Geometry: final body of the model. Coordinates: model frame, mm. A direction names the side the tool comes from. Give positions to 0.01 mm unless a question says otherwise; leave off trailing zeros. Write each loop counter-clockwise with the first axis right and the second up, starting at its lowest first coordinate (ties: lowest second). Pieces come first, ordered by that corner, then holes.
from build123d import *

# Parameters (mm, degrees)
F0_R     = 10.936503
F1_DEPTH = 7.0104
F2_R     = 10.16
F3_R     = 2.54


with BuildPart() as f1:
    # F0 (on Front) → F1 (new body)
    with BuildSketch(Plane.XZ):
        with BuildLine():
            Line((-17.78, 35.56), (-17.78, 10.265288))
            Line((-17.78, 10.265288), (-39.685863, -2.382068))
            ThreePointArc((-39.685863, -2.382068), (-46.193795, -26.67), (-21.905863, -33.177932))
            Line((-21.905863, -33.177932), (0, -20.530576))
            Line((0, -20.530576), (21.905863, -33.177932))
            ThreePointArc((21.905863, -33.177932), (46.193795, -26.67), (39.685863, -2.382068))
            Line((39.685863, -2.382068), (17.78, 10.265288))
            Line((17.78, 10.265288), (17.78, 35.56))
            ThreePointArc((17.78, 35.56), (0, 53.34), (-17.78, 35.56))
        make_face()
        with Locations((-30.795863, -17.78)):
            Circle(F0_R, mode=Mode.SUBTRACT)
        with Locations((30.795863, -17.78)):
            Circle(F0_R, mode=Mode.SUBTRACT)
        Circle(F0_R, mode=Mode.SUBTRACT)
        with Locations((0, 35.56)):
            Circle(F0_R, mode=Mode.SUBTRACT)
    extrude(amount=F1_DEPTH)

    # F2
    f2_edges = [f1.edges().sort_by_distance(p)[0] for p in [
        (17.78, -3.5052, 10.265288),
        (-17.78, -3.5052, 10.265288),
        (0, -3.5052, -20.530576),
    ]]
    fillet(f2_edges, radius=F2_R)

    # F3
    f3_edges = [f1.edges().sort_by_distance(p)[0] for p in [
        (-17.78, -7.0104, 25.845583),
        (-17.78, 0, 25.845583),
    ]]
    fillet(f3_edges, radius=F3_R)


solid = f1.part
Q1. Section C-C on z = 19. Output: boundary loops of the cut face in (x, y).
Filled sheet:
outline: (-17.78, -4.47) arc R2.54 ccw to (-15.24, -7.01) - (15.24, -7.01) arc R2.54 ccw to (17.78, -4.47) - (17.78, -2.54) arc R2.54 ccw to (15.24, 0) - (-15.24, 0) arc R2.54 ccw to (-17.78, -2.54) - close
Q2. Ray query, line 1 along Z through (x, y) = (0, -2.25); line 2 along Z through (x, y) = (9, -2.5); line 3 along Y through (x, z) = (5.5, -21). Return the intervals inside material, ascending.
Filled sheet:
line 1: z = -22.09 to -10.94, 10.94 to 24.62, 46.5 to 53.32
line 2: z = -25.73 to -6.21, 6.21 to 29.35, 41.77 to 50.89
line 3: y = -7 to -0.01
Q3. Section A-A on x = 0. Output: boundary loops of the cut face in (y, z), plus the area to 3 significant figures.
Filled sheet:
outline: (-7.01, -19.56) arc R2.54 ccw to (-4.47, -22.1) - (-2.54, -22.1) arc R2.54 ccw to (0, -19.56) - (0, -10.94) - (-7.01, -10.94) - close; (-7.01, 10.94) - (0, 10.94) - (0, 24.62) - (-7.01, 24.62) - close; (-7.01, 46.5) - (0, 46.5) - (0, 50.8) arc R2.54 ccw to (-2.54, 53.34) - (-4.47, 53.34) arc R2.54 ccw to (-7.01, 50.8) - close
area: 217 mm2
Q4. Section B-B on z = -17.78. Output: boundary loops of the cut face in (x, y), plus the area to 3 significant figures.
Filled sheet:
outline: (-48.58, -4.47) arc R2.54 ccw to (-46.04, -7.01) - (-41.73, -7.01) - (-41.73, 0) - (-46.04, 0) arc R2.54 ccw to (-48.58, -2.54) - close; (-19.86, -7.01) - (19.86, -7.01) - (19.86, 0) - (-19.86, 0) - close; (41.73, -7.01) - (46.04, -7.01) arc R2.54 ccw to (48.58, -4.47) - (48.58, -2.54) arc R2.54 ccw to (46.04, 0) - (41.73, 0) - close
area: 369 mm2
Q5. Pull-direction query (Z, two-part tool) for faces 5 (the cylindrical face through (-1.424, -3.456, 10.843)), 6 (the cylindrical face through (-20.693, -3.456, -21.969)), 7 (the cylindrical face through (0.391, -3.492, 53.336)), 8 (the cylindrical face through (46, -3, -27)); classes: released by +Z, released by -Z, zero draft, split by the parting line, or undercut.
Filled sheet:
face 5: undercut
face 6: undercut
face 7: released by +Z
face 8: split by the parting line
Q6. Access query for faces 1 (the cylindrical face through (17.056, -0.764, 25.982)), 2 (the cylindrical face through (-17.1, -6.2, 25.7)), 3 (the cylindrical face through (-17.056, -0.764, 25.71)), 4 (the flat face through (13.375, -3.492, -28.253)). Directions: +Z, -Z, +X, -X, +Y, -Y. A direction counts if a zero-diameter tool reaches every point of the face in a straight line with its end or side. Return the directions, or none.
Filled sheet:
face 1: +Z, +X, +Y
face 2: +Z, -X, -Y
face 3: +Z, -X, +Y
face 4: -Z, +Y, -Y
Q7. Pin query (flat end, axial travel): P1, Ø0.6, axis at y = -3.5, z = 28.5, coming from the +X side; P2, Ø3, axis at y = -4.5, z = 6.5, coming from the -X side; P3, Ø0.6, axis at y = -3.5, z = 21.5, coming from the -X side. Return the tip coordinate at first contact, or that it passes through.
Filled sheet:
P1: stops at x = 17.78
P2: stops at x = -26.9
P3: stops at x = -17.78
